Here's the drawing with two shaded views (mm, measured from the low corner). I have some questions. Coordinates: 2 decimals unless noted, no trailing zeros. Order: outer loops, then holes, each group sorted by start corner. A loop starts at its lowest first (then second) coordinate and runs counter-clockwise, first axis right, second up. Notation, with made-up numbers: (-28, 67.5) -> (2, 67.5) arc R27 cw to (2, 100.5) -> close; hole circle Ø10 at (74.5, 52). An arc over 180 degrees is marked (long way). Answer in a Markdown table with one row per item. Add a question column.
1. If I drill on line 1 along Y through (x, z) = (12.7, 17.2); line 2 along Z through (x, y) = (11.75, 136.5) (3 decimals); line 3 along X through (y, z) = (201.5, 14) (3 decimals), over which ranges is the centre line in solid material (lowest first)? Write a range as [from, to].
2. Imagine slicing it at B-B on z = 11. Write out the boundary of the cut face in (x, y) (3 decimals), plus the area to 3 significant figures.
3. Will these pins go through, and if not, where does the flat tip stop? pin 1 (5 mm diameter, centred on y = 215.5, z = 11.5, fed in from +X) (3 decimals); pin 2 (8 mm diameter, centred on x = 8, z = 14.5, fed in from -Y); pin 3 (8 mm diameter, centred on x = 10, y = 132.5, fed in from -Z) (3 decimals).
4. Imagine slicing it at A-A on y = 282. Write out the boundary of the cut face in (x, z) (3 decimals).
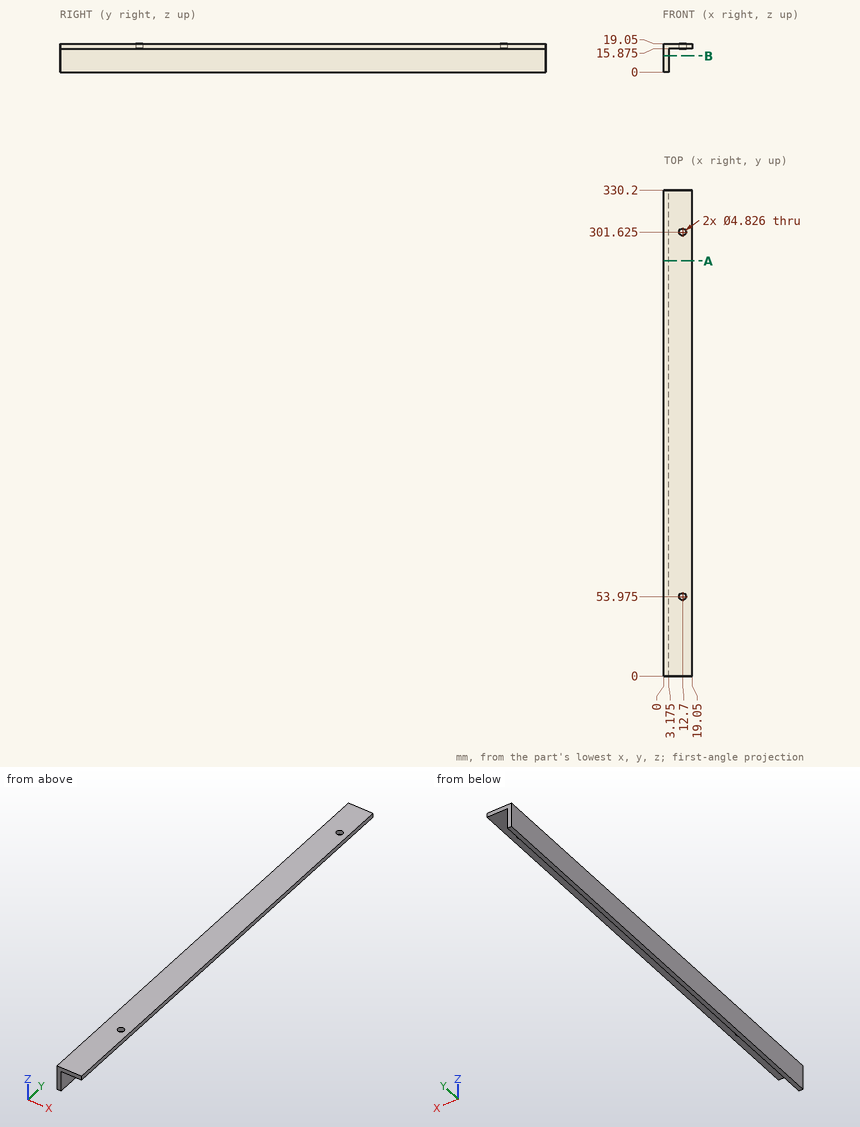
Answers follow:
| question | item | result |
|---|---|---|
| 1 | line 1 | y = [0, 51.56], [56.39, 299.21], [304.04, 330.2] |
| 1 | line 2 | z = [15.875, 19.05] |
| 1 | line 3 | x = [0, 3.175] |
| 2 | outline | (0, 0) -> (3.175, 0) -> (3.175, 330.2) -> (0, 330.2) -> close |
| 2 | area | 1,050 mm² |
| 3 | pin 1 | stops at x = 3.175 |
| 3 | pin 2 | stops at y = 0 |
| 3 | pin 3 | stops at z = 15.875 |
| 4 | outline | (0, 0) -> (3.175, 0) -> (3.175, 15.875) -> (19.05, 15.875) -> (19.05, 19.05) -> (0, 19.05) -> close |
